Verification items for the finished model (mm, model axes). Coordinates: 2 decimals unless noted, no trailing zeros. Write each loop counter-clockwise with the first axis right and the second up, starting at its lowest first coordinate (ties: lowest second). Pieces come first, ordered by that corner, then holes. Notation, with made-up numbers: (17, 48) -> (60, 48) arc R7 cw to (60, 59) -> close; hole circle Ø5 at (28, -2.75). An arc over 180 degrees is marked (long way). Write each question's results on one line, items separated by ' | '. Start each with the question number.
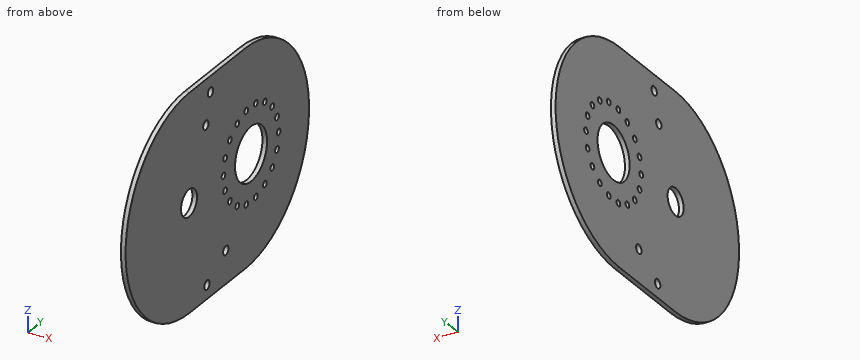
from build123d import *

# Parameters (mm, degrees)
SKETCH1_R           = 29
SKETCH1_R_2         = 14.5
SKETCH1_R_3         = 4.85
BOSS_EXTRUDE1_DEPTH = 5
SCALE1_SCALE        = 1.5
SKETCH2_R           = 5
CUT_EXTRUDE1_DEPTH  = 10


with BuildPart() as part:
    # Sketch1 → Boss-Extrude1 (new body)
    with BuildSketch(Plane(origin=(0, 0, 0), x_dir=(0, 0, -1), z_dir=(1, 0, 0))):
        with BuildLine():
            Line((116, 50.1), (116, -50.1))
            ThreePointArc((116, -50.1), (0, -166.1), (-116, -50.1))
            Line((-116, -50.1), (-116, 50.1))
            ThreePointArc((-116, 50.1), (0, 166.1), (116, 50.1))
        make_face()
        with Locations((0, 61.077179293)):
            Circle(SKETCH1_R, mode=Mode.SUBTRACT)
        with Locations((0, -51.244320707)):
            Circle(SKETCH1_R_2, mode=Mode.SUBTRACT)
        with Locations((80.472730607, 15.380858581)):
            Circle(SKETCH1_R_3, mode=Mode.SUBTRACT)
        with Locations((101.210456573, -18.715580545)):
            Circle(SKETCH1_R_3, mode=Mode.SUBTRACT)
        with Locations((-67.898806967, -20.724176458)):
            Circle(SKETCH1_R_3, mode=Mode.SUBTRACT)
        with Locations((-98.945842281, -12.367503179)):
            Circle(SKETCH1_R_3, mode=Mode.SUBTRACT)
    extrude(amount=BOSS_EXTRUDE1_DEPTH)


with BuildPart() as part_1:
    # Scale1: scaled about (2.5, -2.015956771, 0.017708556)
    add(part.part.scale(SCALE1_SCALE).moved(Location((-1.25, 1.007978385, -0.008854278))))

    # Sketch2 → Cut-Extrude1 (cut)
    with BuildSketch(Plane(origin=(6.25, 0, 0), x_dir=(0, 0, -1), z_dir=(1, 0, 0))):
        with Locations((0.008854278, 167.623747325)):
            Circle(SKETCH2_R)
        with Locations((25.660365027, 163.100693884)):
            Circle(SKETCH2_R)
        with Locations((48.217925004, 150.077080559)):
            Circle(SKETCH2_R)
        with Locations((64.960759562, 130.123747325)):
            Circle(SKETCH2_R)
        with Locations((73.869435754, 105.64736065)):
            Circle(SKETCH2_R)
        with Locations((73.869435754, 79.600134)):
            Circle(SKETCH2_R)
        with Locations((64.960759562, 55.123747325)):
            Circle(SKETCH2_R)
        with Locations((48.217925004, 35.170414091)):
            Circle(SKETCH2_R)
        with Locations((25.660365027, 22.146800766)):
            Circle(SKETCH2_R)
        with Locations((0.008854278, 17.623747325)):
            Circle(SKETCH2_R)
        with Locations((-25.642656472, 22.146800766)):
            Circle(SKETCH2_R)
        with Locations((-48.200216449, 35.170414091)):
            Circle(SKETCH2_R)
        with Locations((-64.943051006, 55.123747325)):
            Circle(SKETCH2_R)
        with Locations((-73.851727198, 79.600134)):
            Circle(SKETCH2_R)
        with Locations((-73.851727198, 105.64736065)):
            Circle(SKETCH2_R)
        with Locations((-64.943051006, 130.123747325)):
            Circle(SKETCH2_R)
        with Locations((-48.200216449, 150.077080559)):
            Circle(SKETCH2_R)
        with Locations((-25.642656472, 163.100693884)):
            Circle(SKETCH2_R)
    extrude(amount=-CUT_EXTRUDE1_DEPTH, mode=Mode.SUBTRACT)


solid = part_1.part
1. Sectioned sample at D-D on z = 135.5. Record the cut outline in (x, y).
2. Sectioned sample at B-B on x = 1.5. State how many separate pieces and enclosed holes the cut face has, plus the area to 3 significant figures.
3. Material ranges on probe 1 along Z at (x, y) = (5.5, 83); probe 2 along Y at (x, z) = (-0.5, -76); probe 3 along Y at (x, z) = (0.5, 27), recorded low to high. Write a range as from..to.
4. Sectioned sample at A-A on y = -89. Record the cut outline in (x, z).
5. Depth check by flat-ended pin: pin 1 Ø8 at (y, z) = (105.65, 73.85) entering from +X; pin 2 Ø11.5 at (y, z) = (163.1, -25.66) entering from +X; pin 3 Ø1 at (x, z) = (5.5, -37) entering from -Y; pin 4 Ø1.5 at (x, z) = (4.5, -113.5) entering from +Y. Enter the tip coordinate at first touch or a pass-through.
6. Sectioned sample at C-C on y = 205.5. Record the cut outline in (x, z).
Computed values:
1) outline: (-1.25, -183.29) -> (6.25, -183.29) -> (6.25, 185.31) -> (-1.25, 185.31) -> close
2) separate pieces: 1 | enclosed holes: 24 | area: 138,000 mm^2
3) probe 1: z = -173.87..-77.54, -70.2..-42.43, 42.41..70.19, 77.52..173.86 | probe 2: y = -230.67..75.08, 84.12..101.12, 110.17..232.69 | probe 3: y = -246.03..17.33, 26.96..58.52, 126.72..158.29, 167.91..248.05
4) outline: (-1.25, -173.37) -> (6.25, -173.37) -> (6.25, -17.34) -> (-1.25, -17.34) -> close; (-1.25, 17.32) -> (6.25, 17.32) -> (6.25, 173.36) -> (-1.25, 173.36) -> close
5) pin 1: passes through | pin 2: stops at x = 6.25 | pin 3: stops at y = -244.27 | pin 4: stops at y = 208.69
6) outline: (-1.25, -116.4) -> (6.25, -116.4) -> (6.25, 116.38) -> (-1.25, 116.38) -> close
